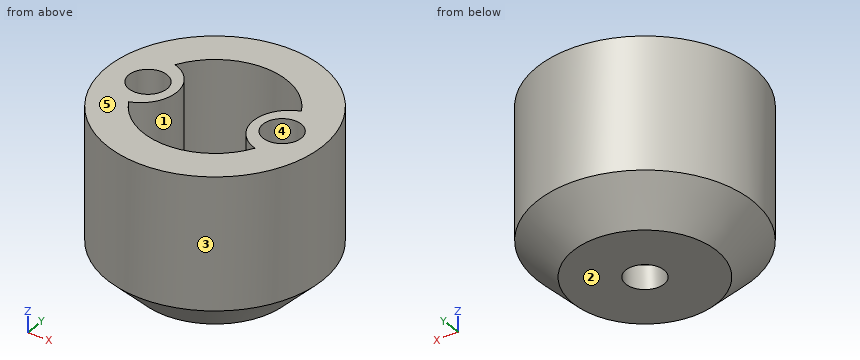
from build123d import *

# Parameters (mm, degrees)
SKETCH006_R       = 4.5
PAD002_DEPTH      = 6
PAD002_DEPTH_BACK = 1
SKETCH007_R       = 3
POCKET008_DEPTH   = 6
SKETCH008_R       = 0.8
HOLE_DEPTH        = 25
PAD005_DEPTH      = 6
SKETCH010_R       = 0.8
POCKET005_DEPTH   = 7
CHAMFER_SIZE      = 1.5


with BuildPart() as part:
    # Sketch006 → Pad002 (new body, two sides)
    with BuildSketch(Plane.XY) as pad002_sk:
        Circle(SKETCH006_R)
    extrude(amount=PAD002_DEPTH)
    extrude(pad002_sk.sketch, amount=-PAD002_DEPTH_BACK)

    # Sketch007 → Pocket008 (cut)
    with BuildSketch(Plane.XY):
        Circle(SKETCH007_R)
    extrude(amount=POCKET008_DEPTH, mode=Mode.SUBTRACT)

    # Sketch008 → Hole (cut)
    with BuildSketch(Plane.XY):
        Circle(SKETCH008_R)
    extrude(amount=-HOLE_DEPTH, mode=Mode.SUBTRACT)

    # Sketch009 → Pad005 (join)
    with BuildSketch(Plane.XY):
        with BuildLine():
            ThreePointArc((-3.1, -1.5), (-1.6, 0), (-3.1, 1.5))
            Line((-3.1, 1.5), (-3.708099, 1.5))
            ThreePointArc((-3.708099, 1.5), (-4, 0), (-3.708099, -1.5))
            Line((-3.1, -1.5), (-3.708099, -1.5))
        make_face()
    pad005 = extrude(amount=PAD005_DEPTH)

    # Sketch010 → Pocket005 (cut)
    with BuildSketch(Plane.XY):
        with Locations((-2.8, 0)):
            Circle(SKETCH010_R)
    pocket005 = extrude(amount=POCKET005_DEPTH, mode=Mode.SUBTRACT)

    # Mirrored005: Pad005, Pocket005 across Sketch009 V_Axis
    add(pad005.mirror(Plane(origin=(0, 0, 0), x_dir=(0, 0, 1), z_dir=(1, 0, 0))))
    add(pocket005.mirror(Plane(origin=(0, 0, 0), x_dir=(0, 0, 1), z_dir=(1, 0, 0))), mode=Mode.SUBTRACT)

    # Chamfer
    chamfer_edges = [part.edges().sort_by_distance(p)[0] for p in [
        (-4.5, 0, -1),
    ]]
    chamfer(chamfer_edges, length=CHAMFER_SIZE)


solid = part.part
Geometry: final body of the model. Coordinates: model frame, mm. Face numbers are marked on the shaded views. A direction names the side the tool comes from. Round coordinates to 2 decimals unless told otherwise and drop trailing zeros. Write each loop counter-clockwise with the first axis right and the second up, starting at its lowest first coordinate (ties: lowest second). Pieces come first, ordered by that corner, then holes. Notation, with made-up numbers: M 81,88 L 89,88 A22 ccw 89,123 Z; hole C 36.5,-13.5 d2. An arc over 180 degrees is marked long. Write item = value, one per line.
Item 1: Section query C-C on y = 0. Return loops of the section in (x, z).
Findings:
outline = M -4.5,0.5 L -3,-1 L -0.8,-1 L -0.8,0 L -1.6,0 L -1.6,6 L -2,6 L -2,0 L -3.6,0 L -3.6,6 L -4.5,6 Z; M 0.8,-1 L 3,-1 L 4.5,0.5 L 4.5,6 L 3.6,6 L 3.6,0 L 2,0 L 2,6 L 1.6,6 L 1.6,0 L 0.8,0 Z
Item 2: Material intervals for line 1 along X through (y, z) = (-1.25, 2.25); line 2 along Y through (x, z) = (-1, 1.25); line 3 along Y through (x, z) = (-2.8, 3.85), sorted ascending. Write a range as [from, to].
Findings:
line_1 = [-4.32, -2.27], [2.27, 4.32]
line_2 = [-4.39, -2.83], [2.83, 4.39]
line_3 = [-3.52, -0.8], [0.8, 3.52]
Item 3: Pull-direction query (Y, two-part tool) for the marked faces 1, 2 and 3; classes: pulls with the +Y half, pulls with the -Y half, needs draft (parallel to the pull), parting line crosses it, or undercut.
Findings:
face_1 = undercut
face_2 = needs draft
face_3 = parting line crosses it
Item 4: Section query A-A on z = 0.25. Return loops of the section in (x, y), then the cut area to 3 significant figures.
Findings:
outline = C 0,0 d8.5; hole C -2.8,0 d1.6; hole M -2.64,-1.43 A3 ccw 2.64,-1.43 A1.5 cw 2.64,1.43 A3 ccw -2.64,1.43 A1.5 cw Z; hole C 2.8,0 d1.6
area = 30.2 mm^2
Item 5: Section query D-D on z = 4.5. Return loops of the section in (x, y), then the cut area to 3 significant figures.
Findings:
outline = C 0,0 d9; hole C -2.8,0 d1.6; hole M -2.64,-1.43 A3 ccw 2.64,-1.43 A1.5 cw 2.64,1.43 A3 ccw -2.64,1.43 A1.5 cw Z; hole C 2.8,0 d1.6
area = 37.1 mm^2
Item 6: Access query for the marked faces 4 and 5. Directions: +Z, -Z, +X, -X, +Y, -Y. A direction counts if a zero-diameter tool reaches every point of the face in a straight line with its end or side. Return the directions, or none.
Findings:
face_4 = +Z
face_5 = +Z, +X, -X, +Y, -Y
Item 7: Pin query (flat end, axial travel): P1, Ø3, axis at x = 0, z = 0, coming from the +Y side; P2, Ø1.5, axis at y = 1, z = 0.5, coming from the +X side; P3, Ø1, axis at y = -1, z = 2.5, coming from the -X side; P4, Ø1.3, axis at x = 2.8, y = 0, coming from the +Z side. Return the tip coordinate at first contact, or that it passes through.
Findings:
P1 = 4.5
P2 = 4.49
P3 = -4.47
P4 = 0
Item 8: Section query B-B on x = 0. Return loops of the section in (y, z).
Findings:
outline = M -4.5,0.5 L -3,-1 L -0.8,-1 L -0.8,0 L -3,0 L -3,6 L -4.5,6 Z; M 0.8,-1 L 3,-1 L 4.5,0.5 L 4.5,6 L 3,6 L 3,0 L 0.8,0 Z
